Can you work these out from the model? Positions are in its coordinate system, mm. A direction names the side the tool comes from. Give positions to 0.01 mm unless a question says otherwise; leave off trailing zeros. Loops run counter-clockwise (first coordinate to the right, second up) from the corner with the lowest first, then second, coordinate; pieces in that order, holes last. Notation, with made-up numbers: (-22, 55) - (-13, 55) arc R30 ccw to (-13, 85) - close; hole circle Ø5 at (42, 3.25). An arc over 180 degrees is marked (long way). Answer in a Markdown table with one row per item.
from build123d import *

# Parameters (mm, degrees)
F0_W     = 76.2
F0_H     = 16.002
F1_DEPTH = 20.574
F3_DEPTH = 20.574
F4_DEPTH = 6.35
F6_DEPTH = 33.274
F8_DEPTH = 33.274


with BuildPart() as f1:
    # F0 (on Front) → F1 (new body)
    with BuildSketch(Plane.XZ):
        Polygon((0, 28.448), (0, 0), (104.648, 0), (76.2, 28.448), align=None)
        with BuildLine():
            ThreePointArc((30.226, 8.636), (24.638, 14.224), (30.226, 19.812))
            Line((30.226, 19.812), (54.102, 19.812))
            ThreePointArc((54.102, 19.812), (59.69, 14.224), (54.102, 8.636))
            Line((54.102, 8.636), (30.226, 8.636))
        make_face(mode=Mode.SUBTRACT)
        with Locations((38.1, 36.449)):
            Rectangle(F0_W, F0_H)
        with Locations((38.1, 52.451)):
            Rectangle(F0_W, F0_H)
        Polygon((0, 88.9), (0, 60.452), (76.2, 60.452), (104.648, 88.9), align=None)
        with BuildLine():
            Line((54.102, 69.088), (30.226, 69.088))
            ThreePointArc((30.226, 69.088), (24.638, 74.676), (30.226, 80.264))
            Line((30.226, 80.264), (54.102, 80.264))
            ThreePointArc((54.102, 80.264), (59.69, 74.676), (54.102, 69.088))
        make_face(mode=Mode.SUBTRACT)
    extrude(amount=F1_DEPTH)

    # F0 (on Front) → F3 (join)
    with BuildSketch(Plane.XZ):
        Polygon((0, 28.448), (0, 0), (104.648, 0), (76.2, 28.448), align=None)
        with BuildLine():
            ThreePointArc((30.226, 8.636), (24.638, 14.224), (30.226, 19.812))
            Line((30.226, 19.812), (54.102, 19.812))
            ThreePointArc((54.102, 19.812), (59.69, 14.224), (54.102, 8.636))
            Line((54.102, 8.636), (30.226, 8.636))
        make_face(mode=Mode.SUBTRACT)
        with Locations((38.1, 36.449)):
            Rectangle(F0_W, F0_H)
        with Locations((38.1, 52.451)):
            Rectangle(F0_W, F0_H)
        Polygon((0, 88.9), (0, 60.452), (76.2, 60.452), (104.648, 88.9), align=None)
        with BuildLine():
            Line((54.102, 69.088), (30.226, 69.088))
            ThreePointArc((30.226, 69.088), (24.638, 74.676), (30.226, 80.264))
            Line((30.226, 80.264), (54.102, 80.264))
            ThreePointArc((54.102, 80.264), (59.69, 74.676), (54.102, 69.088))
        make_face(mode=Mode.SUBTRACT)
    extrude(amount=F3_DEPTH)

    # F2 (on face) → F4 (join, symmetric)
    with BuildSketch(Plane.XZ.offset(20.574)):
        Polygon((69.596, 17.526), (69.596, 0), (104.648, 0), (87.122, 17.526), align=None)
        Polygon((69.596, 88.9), (69.596, 71.374), (87.122, 71.374), (104.648, 88.9), align=None)
    extrude(amount=F4_DEPTH, both=True)

    # F5 (on face) → F6 (join)
    with BuildSketch(Plane.XZ.offset(26.924)):
        Polygon((87.122, 17.526), (69.596, 17.526), (69.596, 0), (104.648, 0), align=None)
    extrude(amount=-F6_DEPTH)

    # F7 (on face) → F8 (join)
    with BuildSketch(Plane.XZ.offset(26.924)):
        Polygon((104.648, 88.9), (69.596, 88.9), (69.596, 71.374), (87.122, 71.374), align=None)
    extrude(amount=-F8_DEPTH)


solid = f1.part
Q1. On a 3-axis mill with a long thin cutter (end or side, diameter ignored), from which of +Z, -Z, +X, -X, +Y, -Y can I reach the whole of each face in a straight line? I mean faces 4 (the face through (69.596, -24, 9)), 5 (the face through (78, 3, 17.526)), 6 (the face through (59.69, -10.14, 74.8)). Say none if no direction works.
Checked values:
| item | result |
|---|---|
| face 4 | +Z, -Z, -X, -Y |
| face 5 | +X, -X, +Y |
| face 6 | +Y, -Y |
Q2. If we mould it in two halves opening along X, with no side actions, what happens to faces 1 (the face through (0, -10, 45)), 2 (the face through (42, -10, 69.088)), 3 (the face through (65, -10, 88.9))? For each: released by +X, released by -X, zero draft, split by the parting line, or undercut.
Checked values:
| item | result |
|---|---|
| face 1 | released by -X |
| face 2 | undercut |
| face 3 | zero draft |
Q3. Imagine slicing it at C-C, the plane z = 73. Write out the boundary of the cut face in (x, y).
Checked values:
| item | result |
|---|---|
| outline | (0, -20.57) - (24.9, -20.57) - (24.9, 0) - (0, 0) - close; (59.43, -20.57) - (69.6, -20.57) - (69.6, -26.92) - (88.75, -26.92) - (88.75, 6.35) - (69.6, 6.35) - (69.6, 0) - (59.43, 0) - close |
Q4. For pin 1 (3 mm diameter, centred on y = 4.5, z = 10.5, fed in from -X); pin 2 (1 mm diameter, centred on y = 1.5, z = 23.5, fed in from -X); pin 3 (6 mm diameter, centred on x = 22.5, z = 19.5, fed in from -Y); pin 4 (3 mm diameter, centred on y = -4, z = 51.5, fed in from +X), each with a flat end and sliding along its axis, tell me the tip position at first contact or that it passes through.
Checked values:
| item | result |
|---|---|
| pin 1 | stops at x = 69.6 |
| pin 2 | passes through |
| pin 3 | stops at y = -20.57 |
| pin 4 | stops at x = 76.2 |
Q5. Imagine slicing it at B-B, the plane y = -17. Write out the boundary of the cut face in (x, z).
Checked values:
| item | result |
|---|---|
| outline | (0, 0) - (104.65, 0) - (76.2, 28.45) - (76.2, 60.45) - (104.65, 88.9) - (0, 88.9) - close; hole (30.23, 8.64) - (54.1, 8.64) arc R5.59 ccw to (54.1, 19.81) - (30.23, 19.81) arc R5.59 ccw to start; hole (30.23, 69.09) - (54.1, 69.09) arc R5.59 ccw to (54.1, 80.26) - (30.23, 80.26) arc R5.59 ccw to start |
Q6. Imagine slicing it at D-D, the plane x = 94.5. Write out the boundary of the cut face in (y, z).
Checked values:
| item | result |
|---|---|
| outline | (-26.92, 0) - (6.35, 0) - (6.35, 10.15) - (-26.92, 10.15) - close; (-26.92, 78.75) - (6.35, 78.75) - (6.35, 88.9) - (-26.92, 88.9) - close |
Q7. If I drill on line 1 (Z direction, x = 29.5, y = -16); line 2 (X direction, y = -7.5, z = 51); line 3 (Y direction, x = 66.5, z = 49.5), over which ranges is the centre line in solid material (lowest first)? Write a range as [from, to].
Checked values:
| item | result |
|---|---|
| line 1 | z = [0, 8.68], [19.76, 69.14], [80.22, 88.9] |
| line 2 | x = [0, 76.2] |
| line 3 | y = [-20.57, 0] |
Q8. Imagine slicing it at A-A, the plane x = 34. Write out the boundary of the cut face in (y, z), and give its area (3 significant figures).
Checked values:
| item | result |
|---|---|
| outline | (-20.57, 0) - (0, 0) - (0, 8.64) - (-20.57, 8.64) - close; (-20.57, 19.81) - (0, 19.81) - (0, 69.09) - (-20.57, 69.09) - close; (-20.57, 80.26) - (0, 80.26) - (0, 88.9) - (-20.57, 88.9) - close |
| area | 1,370 mm² |
